Design review of the part built by this model. Coordinates are the model's own, in mm. Face numbers are marked on the shaded views. A direction names the side the tool comes from. Give positions to 0.01 mm unless a question says otherwise; leave off trailing zeros. Order: outer loops, then holes, each group sorted by start corner. A loop starts at its lowest first (then second) coordinate and runs counter-clockwise, first axis right, second up.
```python
from build123d import *

# Parameters (mm, degrees)
BASE_FLANGE1_DEPTH  = 41
SKETCH2_W           = 42
SKETCH2_H           = 20
CUT_EXTRUDE1_DEPTH  = 10
BOSS_EXTRUDE1_DEPTH = 6
SKETCH5_R           = 1
CUT_EXTRUDE3_DEPTH  = 165.132308696


# Sheet-metal steps are written as plain solids
with BuildPart() as part:
    # Sketch1 → Base-Flange1 (new body)
    with BuildSketch(Plane(origin=(0, 0, 0), x_dir=(1, 0, 0), z_dir=(0, 1, 0))):
        with BuildLine():
            Line((0, 0), (29.484227127, 0))
            ThreePointArc((29.484227127, 0), (29.90672353, 0.133212604), (30.176404712, 0.484667962))
            Line((30.176404712, 0.484667962), (38.681704054, 23.85278585))
            ThreePointArc((38.681704054, 23.85278585), (40.049733788, 25.635636911), (42.1929595, 26.311393382))
            Line((42.1929595, 26.311393382), (78.441184331, 26.311393382))
            ThreePointArc((78.441184331, 26.311393382), (80.843024514, 25.437195048), (82.121016981, 23.223647163))
            Line((82.121016981, 23.223647163), (84.942198964, 7.223929074))
            ThreePointArc((84.942198964, 7.223929074), (85.194131001, 6.787569985), (85.667608355, 6.615238322))
            Line((85.667608355, 6.615238322), (158.049527566, 6.615238322))
            Line((158.049527566, 6.615238322), (158.049527566, 3.615238322))
            Line((158.049527566, 3.615238322), (85.667608355, 3.615238322))
            ThreePointArc((85.667608355, 3.615238322), (83.265768172, 4.489436656), (81.987775705, 6.702984541))
            Line((81.987775705, 6.702984541), (79.166593722, 22.70270263))
            ThreePointArc((79.166593722, 22.70270263), (78.914661685, 23.139061719), (78.441184331, 23.311393382))
            Line((78.441184331, 23.311393382), (42.1929595, 23.311393382))
            ThreePointArc((42.1929595, 23.311393382), (41.770463097, 23.178180778), (41.500781916, 22.82672542))
            Line((41.500781916, 22.82672542), (32.995482574, -0.541392468))
            ThreePointArc((32.995482574, -0.541392468), (31.627452839, -2.324243529), (29.484227127, -3))
            Line((29.484227127, -3), (0, -3))
            Line((0, -3), (0, 0))
        make_face()
    extrude(amount=BASE_FLANGE1_DEPTH)

    # Sketch2 → Cut-Extrude1 (cut)
    with BuildSketch(Plane.XY.offset(-3.615238322)):
        with Locations((125.049527566, 20)):
            Rectangle(SKETCH2_W, SKETCH2_H)
    extrude(amount=-CUT_EXTRUDE1_DEPTH, mode=Mode.SUBTRACT)

    # Sketch3 → Boss-Extrude1 (add)
    with BuildSketch(Plane.XY.offset(-3.615238322)):
        Polygon((104.049527566, 30), (104.049527566, 41), (92.049527566, 41), (92.049527566, 0), (104.049527566, 0), (104.049527566, 10), align=None)
        Polygon((158.049527566, 0), (158.049527566, 41), (146.049527566, 41), (146.049527566, 30), (146.049527566, 10), (146.049527566, 0), align=None)
    extrude(amount=-BOSS_EXTRUDE1_DEPTH)

    # Sketch5 → Cut-Extrude3 (cut, through all)
    with BuildSketch(Plane(origin=(0, 0, -9.615238322), x_dir=(-1, 0, 0), z_dir=(0, 0, -1))):
        with Locations((-100.049527566, 25)):
            Circle(SKETCH5_R)
        with Locations((-100.049527566, 15)):
            Circle(SKETCH5_R)
        with Locations((-150.049527566, 15)):
            Circle(SKETCH5_R)
        with Locations((-150.049527566, 25)):
            Circle(SKETCH5_R)
    extrude(amount=-CUT_EXTRUDE3_DEPTH, mode=Mode.SUBTRACT)


solid = part.part
```
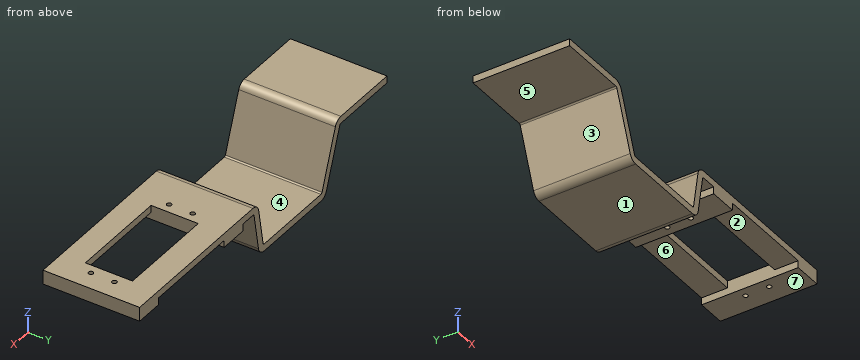
1. Machinability: for the marked faces 4, 5, 6 and 7, which of the approach directions +Z, -Z, +X, -X, +Y, -Y give a long, thin tool a straight path to every point of the face, cutting with its end or side? Answer none if there is none.
Recorded:
face 4: +Z, +Y, -Y
face 5: -Z, -X, +Y, -Y
face 6: -Z, +Y, -Y
face 7: -Z, +X, +Y, -Y
2. Draft analysis for pull direction X (two halves, no side actions). For the marked faces 1, 2 and 3, state which applies: pulls with the +X half, pulls with the -X half, needs draft (parallel to the pull), parting line crosses it, or undercut.
Recorded:
face 1: needs draft
face 2: undercut
face 3: pulls with the -X half
3. Take a section at D-D (y = 36). State the section outline as (x, z) points, then the cut area to 3 significant figures.
Recorded:
outline: (0, 0) - (29.48, 0) arc R0.74 cw to (30.18, -0.48) - (38.68, -23.85) arc R3.74 ccw to (42.19, -26.31) - (78.44, -26.31) arc R3.74 ccw to (82.12, -23.22) - (84.94, -7.22) arc R0.74 cw to (85.67, -6.62) - (92.05, -6.62) - (92.05, -9.62) - (104.05, -9.62) - (104.05, -6.62) - (146.05, -6.62) - (146.05, -9.62) - (158.05, -9.62) - (158.05, -3.62) - (85.67, -3.62) arc R3.74 ccw to (81.99, -6.7) - (79.17, -22.7) arc R0.74 cw to (78.44, -23.31) - (42.19, -23.31) arc R0.74 cw to (41.5, -22.83) - (33, 0.54) arc R3.74 ccw to (29.48, 3) - (0, 3) - close
area: 645 mm2
4. Take a section at C-C (z = -12). State the section outline as (x, y) points.
Recorded:
outline: (34.37, 0) - (37.56, 0) - (37.56, 41) - (34.37, 41) - close; (81.05, 0) - (84.1, 0) - (84.1, 41) - (81.05, 41) - close
5. For pin 1 (9.5 mm diameter, centred on x = 96, y = 29, fed in from -Z); pin 2 (4 mm diameter, centred on x = 141, y = 33.5, fed in from +Z); pin 3 (1.6 mm diameter, centred on x = 150.05, y = 25, fed in from +Z); pin 4 (10 mm diameter, centred on y = 14, z = -20, fed in from +X), all flat-tipped, find the tip position at first contact; note any pin that passes through.
Recorded:
pin 1: stops at z = -9.62
pin 2: stops at z = -3.62
pin 3: passes through
pin 4: stops at x = 83.57
6. For line 1 along X through (y, z) = (13, -9); line 2 along Z through (x, y) = (87, 6); line 3 along Z through (x, y) = (58.5, 37), list the stretches that pass through material, from the lowest coordinate up.
Recorded:
line 1: x = 33.28 to 36.47, 81.58 to 84.63, 92.05 to 104.05, 146.05 to 158.05
line 2: z = -6.62 to -3.62
line 3: z = -26.31 to -23.31
7. Take a section at A-A (x = 132.5). State the section outline as (y, z) points.
Recorded:
outline: (0, -6.62) - (10, -6.62) - (10, -3.62) - (0, -3.62) - close; (30, -6.62) - (41, -6.62) - (41, -3.62) - (30, -3.62) - close
8. Take a section at B-B (y = 21). State the section outline as (x, z) points.
Recorded:
outline: (0, 0) - (29.48, 0) arc R0.74 cw to (30.18, -0.48) - (38.68, -23.85) arc R3.74 ccw to (42.19, -26.31) - (78.44, -26.31) arc R3.74 ccw to (82.12, -23.22) - (84.94, -7.22) arc R0.74 cw to (85.67, -6.62) - (92.05, -6.62) - (92.05, -9.62) - (104.05, -9.62) - (104.05, -3.62) - (85.67, -3.62) arc R3.74 ccw to (81.99, -6.7) - (79.17, -22.7) arc R0.74 cw to (78.44, -23.31) - (42.19, -23.31) arc R0.74 cw to (41.5, -22.83) - (33, 0.54) arc R3.74 ccw to (29.48, 3) - (0, 3) - close; (146.05, -9.62) - (158.05, -9.62) - (158.05, -3.62) - (146.05, -3.62) - close
